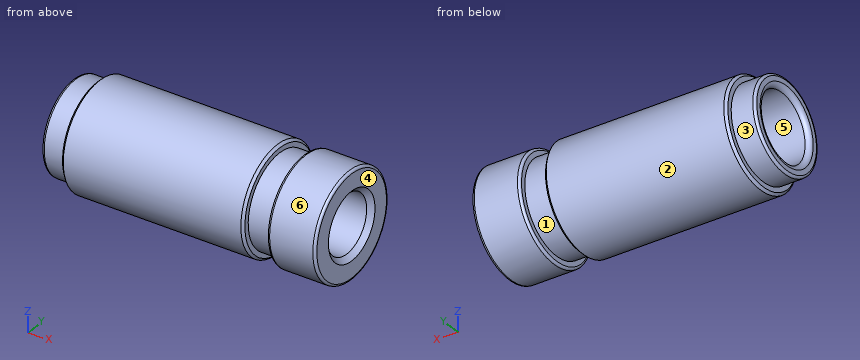
```python
from build123d import *

# Parameters (mm, degrees)
ESBO_O2_R                        = 7
CORTE_EXTRUS_O1_DEPTH            = 25
FURO_ROSCADO_DE_M141_D           = 12
FURO_ROSCADO_DE_M141_DEPTH       = 35
FURO_ROSCADO_DE_M141_CSINK_D     = 14.05
FURO_ROSCADO_DE_M141_CSINK_ANGLE = 90
FURO_ROSCADO_DE_M141_TIP         = 3.605163714
FILETE1_R                        = 0.5
FILETE2_R                        = 1
CHANFRO1_SIZE                    = 0.5


with BuildPart() as part:
    # Esboço1 → Revolução1 (revolve)
    with BuildSketch(Plane.XY, mode=Mode.PRIVATE) as revolu_o1_sk:
        Polygon((0, 0), (58, 0), (58, 11), (48, 11), (48, 9.5), (43, 9.5), (43, 11), (5, 11), (5, 9.5), (0, 9.5), align=None)
    revolve(revolu_o1_sk.sketch.rotate(Axis((0, 0, 0), (1, 0, 0)), 90), axis=Axis((0, 0, 0), (1, 0, 0)))

    # Esboço2 → Corte-extrusão1 (cut)
    with BuildSketch(Plane.ZY):
        Circle(ESBO_O2_R)
    extrude(amount=-CORTE_EXTRUS_O1_DEPTH, mode=Mode.SUBTRACT)

    # Furo roscado de M141
    with Locations(Plane(origin=(58, 0, 0), x_dir=(0, 0, -1), z_dir=(1, 0, 0))):
        with Locations((0, 0)):
            CounterSinkHole(FURO_ROSCADO_DE_M141_D / 2, FURO_ROSCADO_DE_M141_CSINK_D / 2, depth=FURO_ROSCADO_DE_M141_DEPTH, counter_sink_angle=FURO_ROSCADO_DE_M141_CSINK_ANGLE)
            with Locations((0, 0, -(FURO_ROSCADO_DE_M141_DEPTH + FURO_ROSCADO_DE_M141_TIP / 2))):  # 118° drill point
                Cone(0, FURO_ROSCADO_DE_M141_D / 2, FURO_ROSCADO_DE_M141_TIP, mode=Mode.SUBTRACT)

    # Filete1
    filete1_edges = [part.edges().sort_by_distance(p)[0] for p in [
        (58, 0, -11),
        (0, 0, -9.5),
        (48, 0, -11),
    ]]
    fillet(filete1_edges, radius=FILETE1_R)

    # Filete2
    filete2_edges = [part.edges().sort_by_distance(p)[0] for p in [
        (0, 0, -7),
    ]]
    fillet(filete2_edges, radius=FILETE2_R)

    # Chanfro1
    chanfro1_edges = [part.edges().sort_by_distance(p)[0] for p in [
        (5, 0, -11),
        (43, 0, -11),
    ]]
    chamfer(chanfro1_edges, length=CHANFRO1_SIZE)


solid = part.part
```
Could you check a few things on this model? Use its own coordinates, in mm. Face numbers are marked on the shaded views. A direction names the side the tool comes from. Coordinates: 2 decimals unless noted, no trailing zeros. Order: outer loops, then holes, each group sorted by start corner. A loop starts at its lowest first (then second) coordinate and runs counter-clockwise, first axis right, second up. Notation, with made-up numbers: M 22.25,25 L 61.25,25 A23 cw 61.25,44 Z; hole C 78,47 d8. An arc over 180 degrees is marked long. Use one line per item in the form item = value. Start each with the question number.
1. We'd pull the mould along Y, two halves only. Please class the marked faces 4, 5 and 6: +Y half, -Y half, draft (parallel to the pull), parting line (faces both ways), or undercut.
2. Please list where these lines run through material, in increasing order: line 1 (Y direction, x = 12, z = 0); line 2 (X direction, y = 6.25, z = 7.25); line 3 (Y direction, x = 37.5, z = 0).
3. Suppose I cut it at A-A on x = 28.5. Write out the boundary of the cut face in (y, z), then the cut area to 3 significant figures.
4. Suppose I cut it at B-B on x = 7.5. Write out the boundary of the cut face in (y, z).
5. For pin 1 (12 mm diameter, centred on x = 43, z = 5, fed in from +Y); pin 2 (3 mm diameter, centred on x = 10, y = 5, fed in from +Z); pin 3 (1.5 mm diameter, centred on x = 49.5, z = 5, fed in from -Y); pin 4 (10 mm diameter, centred on x = 20, z = 6, fed in from -Y), each with a flat end and sliding along its axis, tell me the tip position at first contact or that it passes through.
6. On a 3-axis mill with a long thin cutter (end or side, diameter ignored), from which of +Z, -Z, +X, -X, +Y, -Y can I reach the whole of each face in a straight line? I mean the marked faces 1, 2 and 3. Say none if no direction works.
Geometry says:
q1.face_4 = draft
q1.face_5 = undercut
q1.face_6 = parting line
q2.line_1 = -11 to -7, 7 to 11
q2.line_2 = 5 to 43, 48 to 58
q2.line_3 = -11 to -6, 6 to 11
q3.outline = C 0,0 d22; hole C 0,0 d12
q3.area = 267 mm^2
q4.outline = C 0,0 d22; hole C 0,0 d14
q5.pin_1 = 11
q5.pin_2 = 10.43
q5.pin_3 = -10.15
q5.pin_4 = -10.95
q6.face_1 = none
q6.face_2 = +X, -X
q6.face_3 = -X
